Source: CAD feature listing. Evaluate the final solid. Frame: model axes, mm. Round coordinates to 2 decimals unless told otherwise and drop trailing zeros. Loops run counter-clockwise (first coordinate to the right, second up) from the corner with the lowest first, then second, coordinate; pieces in that order, holes last. Notation, with made-up numbers: (53, 47) -> (90, 47) arc R30 cw to (90, 80) -> close; hole circle Ø5 at (-3.75, 81). An arc over 180 degrees is marked (long way). Return JSON: item names as keys, results as strings. Group by question number.
```python
from build123d import *

# Parameters (mm, degrees)
SKETCH1_R           = 15
BOSS_EXTRUDE1_DEPTH = 590
BOSS_EXTRUDE3_START = -55
BOSS_EXTRUDE3_DEPTH = 55
BOSS_EXTRUDE4_DEPTH = 40


with BuildPart() as part:
    # Sketch1 → Boss-Extrude1 (new body)
    with BuildSketch(Plane(origin=(0, 0, 0), x_dir=(0, 0, -1), z_dir=(1, 0, 0))):
        Circle(SKETCH1_R)
    extrude(amount=BOSS_EXTRUDE1_DEPTH)

    # Sketch2 → Boss-Extrude3 (add)
    with BuildSketch(Plane(origin=(590, 0, 0), x_dir=(0, 0, -1), z_dir=(1, 0, 0)).offset(BOSS_EXTRUDE3_START)):
        with BuildLine():
            Line((5, 14.142135624), (5, 18.302135624))
            Line((5, 18.302135624), (-5, 18.302135624))
            Line((-5, 18.302135624), (-5, 14.142135624))
            ThreePointArc((-5, 14.142135624), (0, 15), (5, 14.142135624))
        make_face()
    extrude(amount=BOSS_EXTRUDE3_DEPTH)

    # Sketch3 → Boss-Extrude4 (add)
    with BuildSketch(Plane(origin=(590, 0, 0), x_dir=(0, 0, -1), z_dir=(1, 0, 0))):
        with BuildLine():
            Line((-5, 18.302135624), (-5, 14.142135624))
            ThreePointArc((-5, 14.142135624), (0, -15), (5, 14.142135624))
            Line((5, 14.142135624), (5, 18.302135624))
            Line((5, 18.302135624), (-5, 18.302135624))
        make_face()
    extrude(amount=BOSS_EXTRUDE4_DEPTH)


solid = part.part
```
(1) Cut plane C-C (x = 555.5). Return loops of the section in (y, z).
(2) Cut plane B-B (y = 9). Return loops of the section in (x, z), and give its area (3 significant figures).
(3) Cut plane D-D (x = 159.5). Return loops of the section in (y, z).
(4) Pin query (flat end, axial travel): pin 1 (4 mm diameter, centred on x = 227, y = 3, fed in from -Z); pin 2 (1 mm diameter, centred on x = 315.5, z = 3, fed in from -Y); pin 3 (3 mm diameter, centred on x = 182.5, z = 9.5, fed in from +Y). Return the tip coordinate at first contact, or that it passes through.
(5) Ray query, line 1 (Z direction, x = 439, y = -1.5); line 2 (Y direction, x = 513, z = 0); line 3 (Z direction, x = 29, y = -1). Return the intervals inside material, ascending.
(6) Cut plane A-A (z = 0). Return loops of the section in (x, y), and give its area (3 significant figures).
Answers follow:
{
 "1": {"outline": "(14.14, -5) -> (18.3, -5) -> (18.3, 5) -> (14.14, 5) arc R15 ccw (long way) to start"},
 "2": {"outline": "(0, -12) -> (630, -12) -> (630, 12) -> (0, 12) -> close", "area": "15,100 mm^2"},
 "3": {"outline": "circle Ø30 at (0, 0)"},
 "4": {"pin 1": "z = -14.97", "pin 2": "y = -14.79", "pin 3": "y = 12.69"},
 "5": {"line 1": "-14.92 to 14.92", "line 2": "-15 to 15", "line 3": "-14.97 to 14.97"},
 "6": {"outline": "(0, -15) -> (630, -15) -> (630, 18.3) -> (535, 18.3) -> (535, 15) -> (0, 15) -> close", "area": "19,200 mm^2"}
}
